Verification items for the finished model (mm, model axes). Face numbers are marked on the shaded views. A direction names the side the tool comes from. Round coordinates to 2 decimals unless told otherwise and drop trailing zeros. Loops run counter-clockwise (first coordinate to the right, second up) from the corner with the lowest first, then second, coordinate; pieces in that order, holes last. Notation, with made-up numbers: M 82.5,-33 L 97.5,-33 A28 cw 97.5,6 Z; hole C 23.5,21 d11. An arc over 180 degrees is marked long. One line per item, written item: value.
from build123d import *

# Parameters (mm, degrees)
SKETCH_1_R      = 3.5
EXTRUDE_1_DEPTH = 6
EXTRUDE_START   = -40
EXTRUDE_2_DEPTH = 40


with BuildPart() as part:
    # Sketch 1 → Extrude 1 (new body)
    # profile 1 of 2: a face of its own
    with BuildSketch(Plane.XY):
        with BuildLine():
            ThreePointArc((-19.861209285, -1.436174734), (-17.268578902, -5.788838852), (-12.5, -7.5))
            Line((-12.5, -7.5), (12.5, -7.5))
            ThreePointArc((12.5, -7.5), (17.268578902, -5.788838852), (19.861209285, -1.436174734))
            Line((19.861209285, -1.436174734), (25, 24.903039453))
            Line((25, 24.903039453), (25, 32.306078854))
            ThreePointArc((25, 32.306078854), (22.769312351, 27.065347755), (17.5, 24.903039453))
            Line((17.5, 24.903039453), (-17.5, 24.903039453))
            ThreePointArc((-17.5, 24.903039453), (-22.803300859, 27.099738594), (-25, 32.403039453))
            Line((-25, 32.403039453), (-25, 24.903039453))
            Line((-25, 24.903039453), (-19.861209285, -1.436174734))
        make_face()
        with Locations((-12.5, 0)):
            Circle(SKETCH_1_R, mode=Mode.SUBTRACT)
        with Locations((12.5, 0)):
            Circle(SKETCH_1_R, mode=Mode.SUBTRACT)
    # profile 2 of 2: a face of its own
    with BuildSketch(Plane.XY):
        with BuildLine():
            Line((-25, 34.903039453), (-25, 32.403039453))
            ThreePointArc((-25, 32.403039453), (-22.803300859, 27.099738594), (-17.5, 24.903039453))
            Line((-17.5, 24.903039453), (17.5, 24.903039453))
            ThreePointArc((17.5, 24.903039453), (22.769312351, 27.065347755), (25, 32.306078854))
            Line((25, 32.306078854), (25, 32.5))
            Line((25, 32.5), (25, 34.903039453))
            ThreePointArc((25, 34.903039453), (23.535533906, 38.438573359), (20, 39.903039453))
            Line((20, 39.903039453), (-20, 39.903039453))
            ThreePointArc((-20, 39.903039453), (-23.535533906, 38.438573359), (-25, 34.903039453))
        make_face()
    extrude(amount=EXTRUDE_1_DEPTH)

    # Sketch 1_6 → Extrude 2 (add)
    with BuildSketch(Plane.XY.offset(EXTRUDE_START)):
        with BuildLine():
            Line((-25, 34.903039453), (-25, 32.403039453))
            ThreePointArc((-25, 32.403039453), (-22.803300859, 27.099738594), (-17.5, 24.903039453))
            Line((-17.5, 24.903039453), (17.5, 24.903039453))
            ThreePointArc((17.5, 24.903039453), (22.769312351, 27.065347755), (25, 32.306078854))
            Line((25, 32.306078854), (25, 32.5))
            Line((25, 32.5), (25, 34.903039453))
            ThreePointArc((25, 34.903039453), (23.535533906, 38.438573359), (20, 39.903039453))
            Line((20, 39.903039453), (-20, 39.903039453))
            ThreePointArc((-20, 39.903039453), (-23.535533906, 38.438573359), (-25, 34.903039453))
        make_face()
    extrude(amount=EXTRUDE_2_DEPTH)


solid = part.part
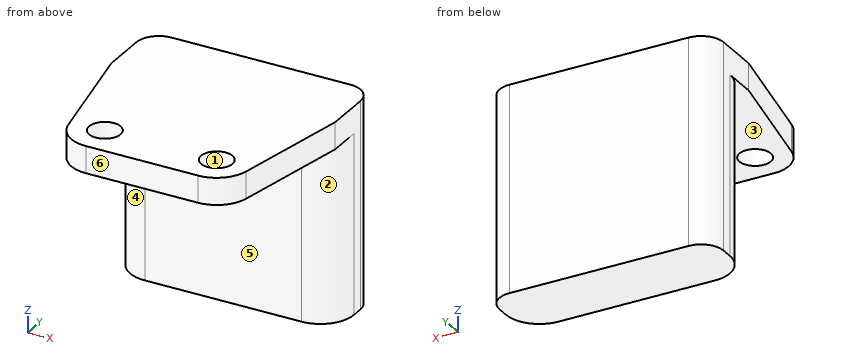
(1) Mould release check, pull along Y, two halves, no side actions. Record for the marked faces 1, 2 and 3: +Y half, -Y half, draft (parallel to the pull), parting line (faces both ways), or undercut.
Completed:
face 1: undercut
face 2: -Y half
face 3: draft
(2) Depth check by flat-ended pin: pin 1 Ø9 at (x, y) = (12.5, 0) entering from -Z; pin 2 Ø8 at (x, z) = (8, -17) entering from -Y; pin 3 Ø6 at (y, z) = (28.5, -23) entering from -X; pin 4 Ø5.5 at (x, y) = (-12.5, 0) entering from +Z. Enter the tip coordinate at first touch or a pass-through.
Completed:
pin 1: stops at z = 0
pin 2: stops at y = 24.9
pin 3: stops at x = -24.95
pin 4: passes through
(3) Sectioned sample at C-C on y = 0. Enter the section's corners in (x, z).
Completed:
outline: M -20.14,0 L -16,0 L -16,6 L -20.14,6 Z; M -9,0 L 9,0 L 9,6 L -9,6 Z; M 16,0 L 20.14,0 L 20.14,6 L 16,6 Z
(4) Tool access check on the marked faces 4, 5 and 6. Record the directions out of +Z, -Z, +X, -X, +Y, -Y that give a thin tool (end or side, any length) a straight path to the whole face; none if there is none.
Completed:
face 4: -Z, -X, -Y
face 5: -Z, +X, -X, -Y
face 6: +Z, -Z, +X, -X, -Y
(5) Sectioned sample at A-A on z = 1.5. Enter the section's corners in (x, y).
Completed:
outline: M -25,24.9 L -19.86,-1.44 A7.5 ccw -12.5,-7.5 L 12.5,-7.5 A7.5 ccw 19.86,-1.44 L 25,24.9 L 25,34.9 A5 ccw 20,39.9 L -20,39.9 A5 ccw -25,34.9 Z; hole C -12.5,0 d7; hole C 12.5,0 d7
(6) Sectioned sample at D-D on z = -19.5. Enter the section's corners in (x, y).
Completed:
outline: M -25,32.4 A7.5 ccw -17.5,24.9 L 17.5,24.9 A7.5 ccw 25,32.31 L 25,34.9 A5 ccw 20,39.9 L -20,39.9 A5 ccw -25,34.9 Z
(7) Thickness scan on L1, parallel to Y at x = 12.5, z = 3.3; L2, parallel to Y at x = -2.5, z = -22; L3, parallel to Z at x = 10, y = 20.5. Record the ranges inside material, lowest first. Write a range as from..to.
Completed:
L1: y = -7.5..-3.5, 3.5..39.9
L2: y = 24.9..39.9
L3: z = 0..6
(8) Sectioned sample at B-B on x = 4. Enter the section's corners in (y, z).
Completed:
outline: M -7.5,0 L 24.9,0 L 24.9,-40 L 39.9,-40 L 39.9,6 L -7.5,6 Z
